Print and shaded views of the part. All mm, measured from the part's lowest x, y and z. Round coordinates to 2 decimals unless told otherwise and drop trailing zeros. Write each loop counter-clockwise with the first axis right and the second up, starting at its lowest first coordinate (ties: lowest second). Pieces come first, ordered by that corner, then holes.
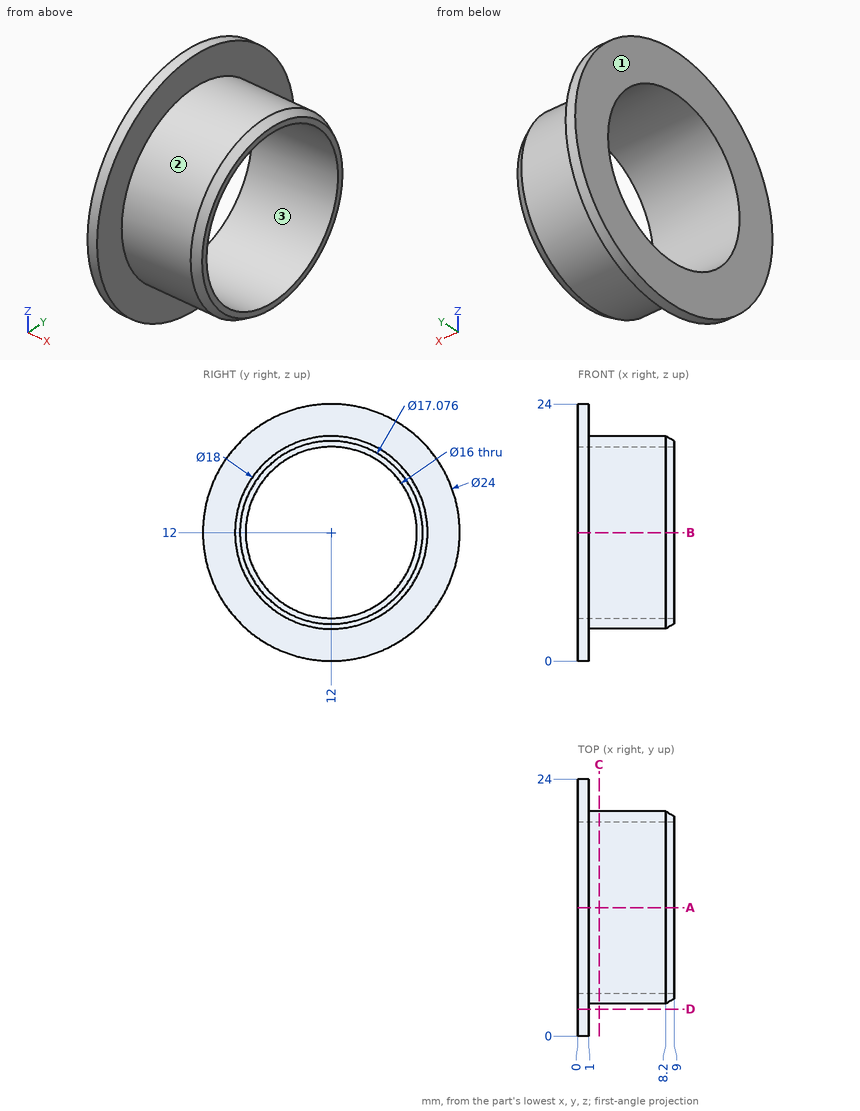
1) Wall check: L1, parallel to Z at x = 5.5, y = 12; L2, parallel to X at y = 21.75, z = 18.5. Give the ranges that are in metal, low to high.
Results:
L1: z = 3 to 4, 20 to 21
L2: x = 0 to 1
2) Slice it at D-D (y = 2.5). Write the cut outline in (x, z).
Results:
outline: (0, 4.67) - (1, 4.67) - (1, 19.33) - (0, 19.33) - close
3) Slice it at C-C (x = 2). Write the cut outline in (y, z).
Results:
outline: circle Ø18 at (12, 12); hole circle Ø16 at (12, 12)
4) Pin check, flat tips, straight feed: pin 1 Ø3 at (x, z) = (3.5, 11.5) entering from +Y; pin 2 Ø13 at (y, z) = (12, 12) entering from -X; pin 3 Ø3 at (x, y) = (7.5, 18) entering from +Z; pin 4 Ø1 at (x, y) = (3, 20) entering from -Z (1 decimal). Stop position of each tip, or through.
Results:
pin 1: stops at y = 21
pin 2: passes through
pin 3: stops at z = 19.79
pin 4: stops at z = 7
5) Mould opens along Z. For the marked faces 1, 2 and 3 say: released by +Z, released by -Z, zero draft, split by the parting line, or undercut.
Results:
face 1: zero draft
face 2: split by the parting line
face 3: undercut
6) Slice it at A-A (y = 12). Write the cut outline in (x, z).
Results:
outline: (0, 0) - (1, 0) - (1, 3) - (8.2, 3) - (9, 3.46) - (9, 4) - (0, 4) - close; (0, 20) - (9, 20) - (9, 20.54) - (8.2, 21) - (1, 21) - (1, 24) - (0, 24) - close
